For this review, use the dimensioned drawing (mm, ordinates from the lowest corner) and the shaded views. A direction names the side the tool comes from. Give positions to 0.01 mm unless a question says otherwise; leave off trailing zeros. Write each loop counter-clockwise with the first axis right and the second up, starting at its lowest first coordinate (ties: lowest second). Pieces come first, ordered by that corner, then holes.
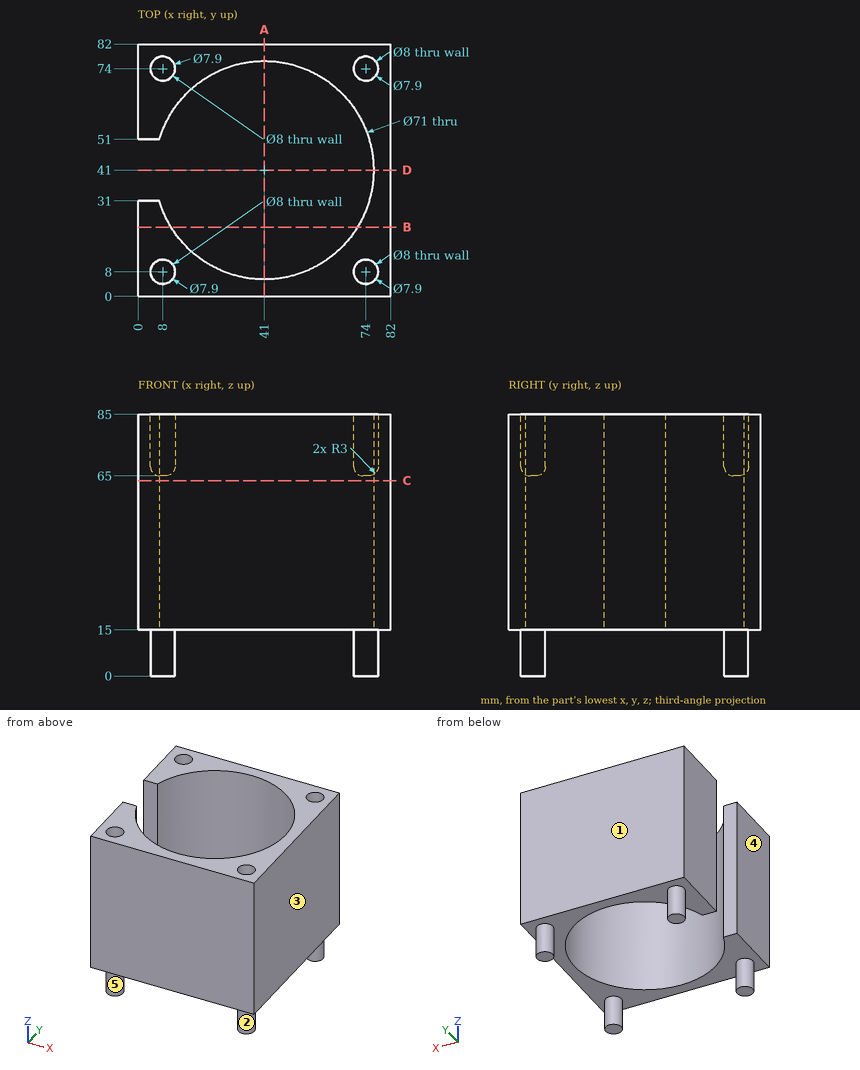
(1) Tool access review of the marked faces 4 and 5: name each direction out of +Z, -Z, +X, -X, +Y, -Y from which nothing blocks a thin tool from reaching the whole face with its end or side.
(2) We need section B-B (y = 22.5). Write out the cut boundary in (x, z), and give its area (3 significant figures).
(3) We need section D-D (y = 41). Write out the cut boundary in (x, z).
(4) The part is to be moulded in two halves that separate along Y. For the marked faces 1, 2 and 3, say which applies: +Y half, -Y half, draft (parallel to the pull), parting line (faces both ways), or undercut.
(5) Clearance check with flat-ended pins moving along their axes: pin 1 Ø2 at (x, y) = (8, 8) entering from +Z; pin 2 Ø24.5 at (x, y) = (30.5, 61) entering from -Z. State where each tip first meets the part, or that it passes through.
(6) We need section A-A (x = 41). Write out the cut boundary in (y, z), and give its area (3 significant figures).
(7) We need section C-C (z = 63.5). Write out the cut boundary in (x, y), and give its area (3 significant figures).
(8) For L1, parallel to Y at x = 74, z = 80.5; L2, parallel to X at y = 42, z = 43; L3, parallel to Z at x = 5, y = 69.5, list the stretches that pass through material, from the lowest coordinate up.
The answers:
1. face 4: +Z, -Z, -X, +Y, -Y
1. face 5: -Z
2. outline: (0, 15) - (10.7, 15) - (10.7, 85) - (0, 85) - close; (71.3, 15) - (82, 15) - (82, 85) - (71.3, 85) - close
2. area: 1,500 mm2
3. outline: (76.5, 15) - (82, 15) - (82, 85) - (76.5, 85) - close
4. face 1: +Y half
4. face 2: undercut
4. face 3: draft
5. pin 1: stops at z = 65
5. pin 2: passes through
6. outline: (0, 15) - (5.5, 15) - (5.5, 85) - (0, 85) - close; (76.5, 15) - (82, 15) - (82, 85) - (76.5, 85) - close
6. area: 770 mm2
7. outline: (0, 0) - (82, 0) - (82, 82) - (0, 82) - (0, 51) - (6.94, 51) arc R35.5 cw (long way) to (6.94, 31) - (0, 31) - close
7. area: 2,650 mm2
8. L1: y = 0 to 4, 12 to 27.91, 54.09 to 70, 78 to 82
8. L2: x = 76.49 to 82
8. L3: z = 15 to 85
